Here's how the part is built. I have some questions about the finished solid (model axes, mm). Face numbers are marked on the shaded views. A direction names the side the tool comes from. Round coordinates to 2 decimals unless told otherwise and drop trailing zeros. Order: outer loops, then holes, each group sorted by start corner. A loop starts at its lowest first (then second) coordinate and runs counter-clockwise, first axis right, second up.
```python
from build123d import *

# Parameters (mm, degrees)
SKETCH1_R           = 26
BOSS_EXTRUDE1_DEPTH = 1.95
SKETCH2_R           = 19
BOSS_EXTRUDE2_DEPTH = 7.25
SKETCH3_R           = 16.5
BOSS_EXTRUDE3_DEPTH = 2.43
SKETCH4_R           = 12.5
BOSS_EXTRUDE4_DEPTH = 8.55
SKETCH5_R           = 7.5
BOSS_EXTRUDE5_DEPTH = 10
SKETCH6_R           = 1.7
BOSS_EXTRUDE6_DEPTH = 10
SKETCH7_R           = 0.85
BOSS_EXTRUDE7_DEPTH = 10
SKETCH8_W           = 3.953217044
SKETCH8_H           = 3.634424256
BOSS_EXTRUDE8_DEPTH = 5


with BuildPart() as part:
    # Sketch1 → Boss-Extrude1 (new body)
    with BuildSketch(Plane.XY):
        Circle(SKETCH1_R)
    extrude(amount=BOSS_EXTRUDE1_DEPTH)

    # Sketch2 → Boss-Extrude2 (add)
    with BuildSketch(Plane(origin=(0, 0, 0), x_dir=(-1, 0, 0), z_dir=(0, 0, -1))):
        Circle(SKETCH2_R)
    extrude(amount=BOSS_EXTRUDE2_DEPTH)

    # Sketch3 → Boss-Extrude3 (add)
    with BuildSketch(Plane.XY.offset(1.95)):
        Circle(SKETCH3_R)
    extrude(amount=BOSS_EXTRUDE3_DEPTH)

    # Sketch4 → Boss-Extrude4 (add)
    with BuildSketch(Plane.XY.offset(4.38)):
        Circle(SKETCH4_R)
    extrude(amount=BOSS_EXTRUDE4_DEPTH)

    # Sketch5 → Boss-Extrude5 (add)
    with BuildSketch(Plane.XY.offset(12.93)):
        Circle(SKETCH5_R)
    extrude(amount=BOSS_EXTRUDE5_DEPTH)

    # Sketch6 → Boss-Extrude6 (add)
    with BuildSketch(Plane(origin=(0, 0, 0), x_dir=(-1, 0, 0), z_dir=(0, 0, -1))):
        with Locations((18.970004687, -12.827662382)):
            Circle(SKETCH6_R)
        with Locations((-20.594083837, -10.014674777)):
            Circle(SKETCH6_R)
        with Locations((1.624079151, 22.84233716)):
            Circle(SKETCH6_R)
    extrude(amount=BOSS_EXTRUDE6_DEPTH)

    # Sketch7 → Boss-Extrude7 (add)
    with BuildSketch(Plane.XY.offset(12.93)):
        with Locations((-10.15, 0)):
            Circle(SKETCH7_R)
        with Locations((-5.075, 8.790157848)):
            Circle(SKETCH7_R)
        with Locations((5.075, 8.790157848)):
            Circle(SKETCH7_R)
        with Locations((10.15, 0)):
            Circle(SKETCH7_R)
        with Locations((5.075, -8.790157848)):
            Circle(SKETCH7_R)
        with Locations((-5.075, -8.790157848)):
            Circle(SKETCH7_R)
    extrude(amount=BOSS_EXTRUDE7_DEPTH)

    # Sketch8 → Boss-Extrude8 (add)
    with BuildSketch(Plane.XY.offset(22.93)):
        Rectangle(SKETCH8_W, SKETCH8_H)
    extrude(amount=BOSS_EXTRUDE8_DEPTH)


solid = part.part
```
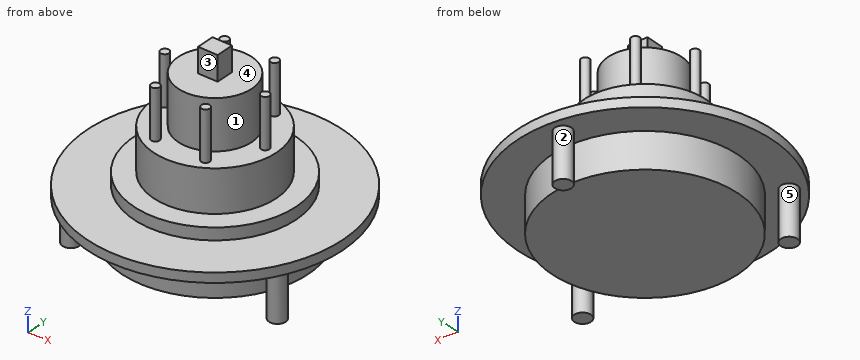
1. I need wall thicknesses on probe 1 along Z at (x, y) = (-15.5, 2); probe 2 along Y at (x, z) = (0, 24); probe 3 along Z at (x, y) = (-14, 12). Which ranges of each line are inside material? Lowest first, please.
Evaluation:
probe 1: z = -7.25 to 4.38
probe 2: y = -1.82 to 1.82
probe 3: z = -7.25 to 1.95
2. If we section it at C-C, the plane x = 14.5: Write out the boundary of the cut face in (y, z), and give its area (3 significant figures).
Evaluation:
outline: (-21.58, 0) - (-12.28, 0) - (-12.28, -7.25) - (12.28, -7.25) - (12.28, 0) - (21.58, 0) - (21.58, 1.95) - (7.87, 1.95) - (7.87, 4.38) - (-7.87, 4.38) - (-7.87, 1.95) - (-21.58, 1.95) - close
area: 300 mm2
3. On a 3-axis mill with a long thin cutter (end or side, diameter ignored), from which of +Z, -Z, +X, -X, +Y, -Y can I reach the whole of each face in a straight line? I mean the marked faces 1 and 2. Say none if no direction works.
Evaluation:
face 1: +Z
face 2: -Z
4. If we section it at D-D, the plane z = 11: Write out the boundary of the cut face in (x, y).
Evaluation:
outline: circle Ø25 at (0, 0)
5. I'm going to push flat-ended pins straight in: P1, Ø1.4, axis at x = -5.5, y = -8.5, coming from the +Z side; P2, Ø1, axis at y = 3, z = 10.5, coming from the +X side; P3, Ø4, axis at x = -10, y = -9.5, coming from the -Z side; P4, Ø20, axis at x = -3, y = 6, coming from the +Z side. Where does each tip first touch, or does it pass through?
Evaluation:
P1: stops at z = 22.93
P2: stops at x = 12.25
P3: stops at z = -7.25
P4: stops at z = 27.93
6. If we section it at B-B, the plane z = 17.5: Write out the boundary of the cut face in (x, y) (3 decimals), and give its area (3 significant figures).
Evaluation:
outline: circle Ø1.7 at (-10.15, 0); circle Ø15 at (0, 0); circle Ø1.7 at (-5.075, -8.79); circle Ø1.7 at (-5.075, 8.79); circle Ø1.7 at (5.075, -8.79); circle Ø1.7 at (5.075, 8.79); circle Ø1.7 at (10.15, 0)
area: 190 mm2
7. If we mould it in two halves opening along Y, with no side actions, what happens to the marked faces 3, 4 and 5? For each: released by +Y, released by -Y, zero draft, split by the parting line, or undercut.
Evaluation:
face 3: released by -Y
face 4: zero draft
face 5: undercut
